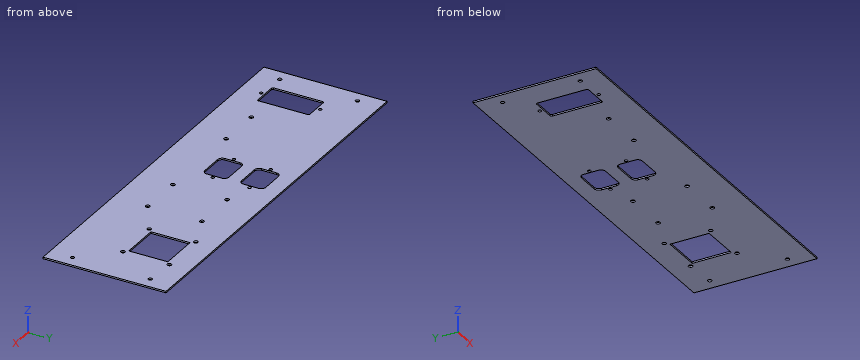
Autodesk Inventor part; units mm, degrees
ref_plane "YZ Plane" through (0, 0, 0) normal (1, 0, 0) x (0, 1, 0)
ref_plane "XZ Plane" through (0, 0, 0) normal (0, 1, 0) x (-1, 0, 0)
ref_plane "XY Plane" through (0, 0, 0) normal (0, 0, 1) x (1, 0, 0)
sketch "Sketch1" plane through (0, 0, 0) normal (0, 0, 1) x (1, 0, 0)
  line L0 (-209.423, -66.294) -> (209.423, -66.294)
  line L1 (209.423, -66.294) -> (209.423, 66.294)
  line L2 (209.423, 66.294) -> (-209.423, 66.294)
  line L3 (-209.423, 66.294) -> (-209.423, -66.294)
  line L4 (-209.423, -66.294) -> (209.423, 66.294) construction
  line L5 (209.423, -66.294) -> (-209.423, 66.294) construction
  point P0 (0, 0)
  dimension "d0" = 418.846
  dimension "d1" = 132.588
extrude "PDU back" add sketch "Sketch1" along normal blind 1.651
sketch "pwr entry" plane through (0, 0, 1.651) normal (0, 0, 1) x (1, 0, 0)
  line L0 (-177.7238, -40.259) -> (-152.2222, -40.259)
  line L1 (-150.6982, -38.735) -> (-150.6982, 14.224)
  line L2 (-152.2222, 15.748) -> (-177.7238, 15.748)
  line L3 (-179.2478, 14.224) -> (-179.2478, -38.735)
  line L4 (-179.2478, -40.259) -> (-150.6982, 15.748) construction
  line L5 (-150.6982, -40.259) -> (-179.2478, 15.748) construction
  line L6 (-164.973, 19.4437) -> (-164.973, -43.9547) construction
  line L7 (-209.423, 66.294) -> (-209.423, -66.294)
  line L8 (-209.423, -66.294) -> (209.423, -66.294)
  arc A0 (-150.6982, 14.224) -> (-152.2222, 15.748) centre (-152.2222, 14.224) ccw
  arc A1 (-177.7238, 15.748) -> (-179.2478, 14.224) centre (-177.7238, 14.224) ccw
  arc A2 (-179.2478, -38.735) -> (-177.7238, -40.259) centre (-177.7238, -38.735) ccw
  arc A3 (-152.2222, -40.259) -> (-150.6982, -38.735) centre (-152.2222, -38.735) ccw
  point P0 (0, 0)
  point P1 (-164.973, -12.2555)
  point P2 (-164.973, -12.2555)
  dimension "d4" = 56.007
  dimension "d5" = 28.5496
  dimension "d6" = 63.3984
  dimension "d7" = 44.45
  dimension "d8" = 22.3393
  dimension "d9" = 1.524
extrude "pwr entry cutout" cut sketch "pwr entry" against normal through all
hole "pwr entry holes" at (-164.973, 19.4437, 1.651) at (-164.973, -43.9547, 1.651) direction (0, 0, -1) diameter 3.4544 end through all
sketch "IEC outlet" plane through (0, 0, 1.651) normal (0, 0, 1) x (1, 0, 0)
  line L0 (-39.116, -16.5735) -> (-4.953, -16.5735)
  line L1 (-4.953, -16.5735) -> (-4.953, 9.4615)
  line L2 (-4.953, 9.4615) -> (-39.116, 9.4615)
  line L3 (-39.116, 9.4615) -> (-39.116, -16.5735)
  line L4 (-39.116, -16.5735) -> (-4.953, 9.4615) construction
  line L5 (-4.953, -16.5735) -> (-39.116, 9.4615) construction
  line L6 (-42.037, -3.556) -> (-2.032, -3.556) construction
  line L7 (-209.423, 66.294) -> (-209.423, -66.294)
  line L8 (-209.423, -66.294) -> (209.423, -66.294)
  line L9 (-39.116, 23.0505) -> (-4.953, 23.0505)
  line L10 (-4.953, 23.0505) -> (-4.953, 49.0855)
  line L11 (-4.953, 49.0855) -> (-39.116, 49.0855)
  line L12 (-39.116, 49.0855) -> (-39.116, 23.0505)
  line L13 (-39.116, 23.0505) -> (-4.953, 49.0855) construction
  line L14 (-4.953, 23.0505) -> (-39.116, 49.0855) construction
  line L15 (-42.037, 36.068) -> (-2.032, 36.068) construction
  point P0 (-22.0345, -3.556)
  point P1 (-22.0345, -3.556)
  point P2 (-22.0345, 36.068)
  point P3 (-22.0345, 36.068)
  dimension "d19" = 26.035
  dimension "d20" = 34.163
  dimension "d22" = 40.005
  dimension "d23" = 167.386
  dimension "d24" = 62.738
  dimension "d129" = 39.624
hole "IEC holes" at (-2.032, -3.556, 1.651) at (-42.037, -3.556, 1.651) at (-2.032, 36.068, 1.651) at (-42.037, 36.068, 1.651) direction (0, 0, -1) diameter 3.4544 end through all
sketch "airflow" plane through (0, 0, 1.651) normal (0, 0, 1) x (1, 0, 0)
  line L0 (-209.423, 66.294) -> (-209.423, -66.294)
  line L1 (-209.423, -66.294) -> (209.423, -66.294)
  line L2 (108.331, -11.303) -> (168.275, -11.303) construction
  line L3 (168.275, -11.303) -> (168.275, 48.641) construction
  line L4 (168.275, 48.641) -> (108.331, 48.641) construction
  line L5 (108.331, 48.641) -> (108.331, -11.303) construction
  line L6 (108.331, -11.303) -> (168.275, 48.641) construction
  line L7 (168.275, -11.303) -> (108.331, 48.641) construction
  line L8 (113.284, -6.35) -> (163.322, -6.35) construction
  line L9 (163.322, -6.35) -> (163.322, 43.688) construction
  line L10 (163.322, 43.688) -> (113.284, 43.688) construction
  line L11 (113.284, 43.688) -> (113.284, -6.35) construction
  line L12 (113.284, -6.35) -> (163.322, 43.688) construction
  line L13 (163.322, -6.35) -> (113.284, 43.688) construction
  line L14 (117.221, -2.413) -> (159.385, -2.413)
  line L15 (159.385, -2.413) -> (159.385, 39.751)
  line L16 (159.385, 39.751) -> (117.221, 39.751)
  line L17 (117.221, 39.751) -> (117.221, -2.413)
  line L18 (117.221, -2.413) -> (159.385, 39.751) construction
  line L19 (159.385, -2.413) -> (117.221, 39.751) construction
  line L20 (209.423, 66.294) -> (-209.423, 66.294)
  point P0 (0, 0)
  point P1 (138.303, 18.669)
  point P2 (138.303, 18.669)
  dimension "d76" = 59.944
  dimension "d77" = 59.944
  dimension "d78" = 50.038
  dimension "d79" = 42.164
  dimension "d123" = 22.606
  dimension "d153" = 322.707
sketch "relay holes" plane through (0, 0, 0) normal (0, 0, -1) x (-1, 0, 0)
  circle A0 centre (2.032, -3.556) radius 1.7272 construction
  line L0 (84.9503, 23.1654) -> (84.9503, -54.0444) construction
  line L1 (-209.423, 66.294) -> (209.423, 66.294)
  line L2 (5.08, 36.068) -> (5.08, -3.9037) construction
  line L3 (150.6982, 14.224) -> (150.6982, -38.735)
  line L4 (72.4662, -29.21) -> (120.2182, -29.21) construction
  point P0 (-28.448, -29.21)
  point P1 (-28.448, 29.21)
  point P2 (-76.2, 29.21)
  point P3 (-76.2, -29.21)
  point P4 (-25.4, -29.21)
  point P5 (2.032, 36.068)
  dimension "d138" = 47.752
  dimension "d139" = 37.084
  dimension "d143" = 58.42
  dimension "d148" = 47.752
  dimension "d149" = 95.504
  dimension "d150" = 30.48
  dimension "d175" = 30.48
  dimension "d176" = 47.752
  dimension "d177" = 30.48
hole "Hole5" at (163.322, 43.688, 1.651) at (113.284, 43.688, 1.651) at (113.284, -6.35, 1.651) at (163.322, -6.35, 1.651) direction (0, 0, -1) diameter 4.4958 end through all
extrude "Extrusion6" cut sketch "airflow" against normal blind 25.4
sketch "bracket" plane through (0, 0, 1.651) normal (0, 0, 1) x (1, 0, 0)
  line L0 (209.423, -66.294) -> (209.423, 66.294) construction
  line L1 (209.423, 54.61) -> (190.373, 54.61) construction
  line L2 (190.373, 54.61) -> (190.373, -54.61) construction
  line L3 (190.373, -54.61) -> (209.423, -54.61) construction
  line L4 (209.423, -54.61) -> (209.423, 54.61) construction
  line L5 (209.423, 66.294) -> (-209.423, 66.294) construction
  line L6 (-209.423, 66.294) -> (-209.423, -66.294) construction
  line L7 (-209.423, 54.61) -> (-190.373, 54.61) construction
  line L8 (-190.373, 54.61) -> (-190.373, -54.61) construction
  line L9 (-190.373, -54.61) -> (-209.423, -54.61) construction
  line L10 (-209.423, -54.61) -> (-209.423, 54.61) construction
  point P0 (0, 0)
  point P1 (196.3674, 41.91)
  point P2 (196.3674, -41.91)
  point P3 (-196.3674, -41.91)
  point P4 (-196.3674, 41.91)
  dimension "d94" = 19.05
  dimension "d95" = 109.22
  dimension "d96" = 11.684
  dimension "d103" = 19.05
  dimension "d104" = 109.22
  dimension "d105" = 11.684
  dimension "d121" = 12.7
  dimension "d122" = 5.9944
  dimension "d161" = 12.7
  dimension "d162" = 12.7
  dimension "d163" = 5.9944
  dimension "d164" = 5.9944
  dimension "d165" = 12.7
  dimension "d166" = 5.9944
hole "bracket holes" at (-196.3674, 41.91, 1.651) at (-196.3674, -41.91, 1.651) at (196.3674, 41.91, 1.651) at (196.3674, -41.91, 1.651) direction (0, 0, -1) diameter 4.2926 end through all
extrude "Extrusion7" cut sketch "IEC outlet" against normal through all
fillet "Fillet3" radius 4.9784 8 edges at (-39.116, 49.0855, 0.8255) (-39.116, 23.0505, 0.8255) (-4.953, 23.0505, 0.8255) (-4.953, 49.0855, 0.8255) (-4.953, 9.4615, 0.8255) (-39.116, 9.4615, 0.8255) (-39.116, -16.5735, 0.8255) (-4.953, -16.5735, 0.8255)
hole "Hole8" at (28.448, 29.21, 0) at (76.2, 29.21, 0) at (76.2, -29.21, 0) at (28.448, -29.21, 0) at (-120.2182, -29.21, 0) at (-72.4662, -29.21, 0) direction (0, 0, 1) diameter 4.4958 end through all
properties part number "PDU_chassis_back"
The listing builds one solid part. Answer for the finished solid, in the listing's coordinates (mm). Coordinates: 2 decimals unless noted, no trailing zeros. Return JSON: item names as keys, results as strings. Group by question number.
(1) Given pin 1 Ø3.5 at (x, y) = (196.37, -41.91) entering from +Z, flat-ended and moving along its own axis, determine where the tip first touches the part or whether it passes through.
(2) Find the intervals of material crossed by probe 1 along X at (y, z) = (-29.21, 1.1); probe 2 along X at (y, z) = (36.5, 0.8) (3 decimals); probe 3 along Y at (x, z) = (-23, 0.7), in increasing order. Write a range as from..to.
(3) A cutting plane is placed at A-A on z = 0.85. Count the separate pieces of the cut face and the enclosed holes in it, and give its area (4 significant figures).
The answers:
{
 "1": {"pin 1": "passes through"},
 "2": {"probe 1": "x = -209.42..-179.25, -150.7..-122.47, -117.97..-74.71, -70.22..26.2, 30.7..73.95, 78.45..209.42", "probe 2": "x = -209.423..-43.709, -40.365..-39.116, -4.953..-3.704, -0.36..117.221, 159.385..209.423", "probe 3": "y = -66.29..-16.57, 9.46..23.05, 49.09..66.29"},
 "3": {"separate pieces": "1", "enclosed holes": "24", "area": "50,150 mm^2"}
}
